Input: dimensioned drawing with shaded views. Units: mm. Origin: part minimum x, y, z. Coordinates: 2 decimals unless noted, no trailing zeros. Order: outer loops, then holes, each group sorted by start corner. A loop starts at its lowest first (then second) coordinate and runs counter-clockwise, first axis right, second up.
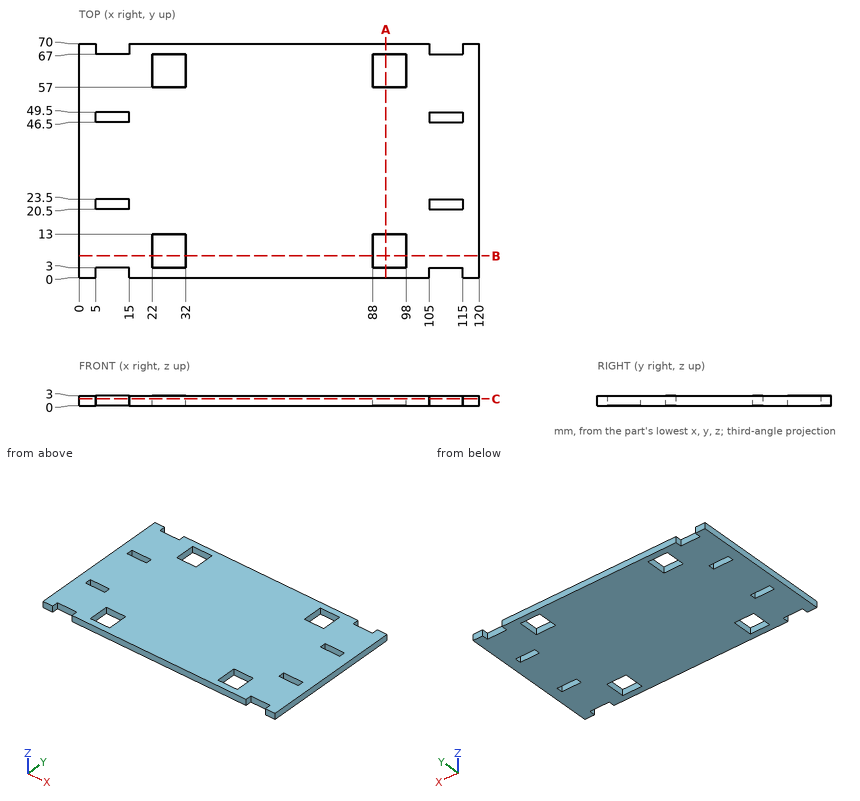
1. Material intervals for line 1 along X through (y, z) = (22, 1.6); line 2 along Y through (x, z) = (10, 1.7); line 3 along X through (y, z) = (7.5, 1.9), sorted ascending.
2. Section query B-B, the plane y = 6.5. Output: boundary loops of the cut face in (x, z), plus the area to 3 significant figures.
3. Contact query for flat-ended pins moving along their axis: P1, Ø1.5, axis at x = 9, z = 1, coming from the -Y side; P2, Ø1.5, axis at x = 9.5, z = 1, coming from the +Y side. Output: stop coordinate, or through.
4. Section query A-A, the plane x = 92. Output: boundary loops of the cut face in (y, z).
5. Section query C-C, the plane z = 2. Count the separate pieces of the cut face and the enclosed holes in it, plus the area to 3 significant figures.
Answer key:
1. line 1: x = 0 to 5, 15 to 105, 115 to 120
1. line 2: y = 3 to 20.5, 23.5 to 46.5, 49.5 to 67
1. line 3: x = 0 to 22, 32 to 88, 98 to 120
2. outline: (0, 0) - (22, 0) - (22, 3) - (0, 3) - close; (32, 0) - (88, 0) - (88, 3) - (32, 3) - close; (98, 0) - (120, 0) - (120, 3) - (98, 3) - close
2. area: 300 mm2
3. P1: stops at y = 3
3. P2: stops at y = 67
4. outline: (0, 0) - (3, 0) - (3, 3) - (0, 3) - close; (13, 0) - (57, 0) - (57, 3) - (13, 3) - close; (67, 0) - (70, 0) - (70, 3) - (67, 3) - close
5. separate pieces: 1
5. enclosed holes: 8
5. area: 7,760 mm2
